Job drawing, mm, ordinate dimensions from the low corner. One solid piece. Round coordinates to 2 decimals unless told otherwise and drop trailing zeros. Loops run counter-clockwise (first coordinate to the right, second up) from the corner with the lowest first, then second, coordinate; pieces in that order, holes last. Notation, with made-up numbers: M 57,-17 L 77,-17 A23 ccw 77,-2 Z; hole C 79.5,52.5 d8. An arc over 180 degrees is marked long. Use a Markdown table: item, result. Add a question column.
(1) Two-plate mould, pull along X, no slides. Class the marked faces 1, 2 and 3: released by +X, released by -X, zero draft, split by the parting line, or undercut.
(2) Band-saw the part on D-D, the plane y = 50.5. Write the cut outline in (x, z).
(3) Wall check: L1, parallel to Y at x = 138.5, z = 4.5; L2, parallel to X at y = 198, z = 8; L3, parallel to X at y = 127, z = 12.25. Give the ranges that are in metal, low to high.
(4) Band-saw the part on A-A, the plane z = 8.5. Give the number of separate pieces and of enclosed holes in the cut face, and give its area (3 significant figures).
(5) Band-saw the part on C-C, the plane y = 127. Write the cut outline in (x, z), and give its area (3 significant figures).
(6) Band-saw the part on B-B, the plane x = 167. Write the cut outline in (y, z), and give its area (3 significant figures).
(7) Flat gauge pins, fed straight in: P1, Ø1.5, axis at y = 228, z = 7.5, coming from the +X side; P2, Ø6, axis at y = 242.5, z = 14.5, coming from the -X side; P3, Ø1, axis at y = 209, z = 14.5, coming from the +X side. Where does each tip first touch, or does it go through?
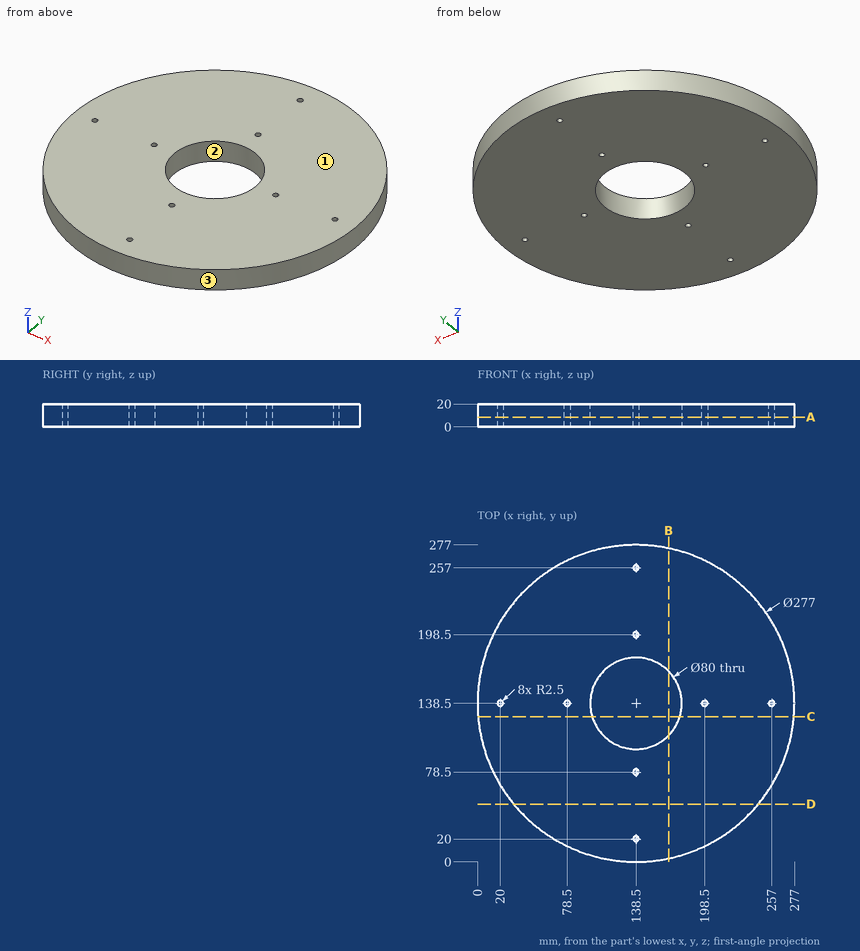
Return value:
| question | item | result |
|---|---|---|
| 1 | face 1 | zero draft |
| 1 | face 2 | undercut |
| 1 | face 3 | split by the parting line |
| 2 | outline | M 31.55,0 L 245.45,0 L 245.45,20 L 31.55,20 Z |
| 3 | L1 | 0 to 17.5, 22.5 to 76, 81 to 98.5, 178.5 to 196, 201 to 254.5, 259.5 to 277 |
| 3 | L2 | 13.43 to 136.05, 140.95 to 263.57 |
| 3 | L3 | 0.48 to 100.19, 176.81 to 276.52 |
| 4 | separate pieces | 1 |
| 4 | enclosed holes | 9 |
| 4 | area | 55,100 mm^2 |
| 5 | outline | M 0.48,0 L 100.19,0 L 100.19,20 L 0.48,20 Z; M 176.81,0 L 276.52,0 L 276.52,20 L 176.81,20 Z |
| 5 | area | 3,990 mm^2 |
| 6 | outline | M 2.96,0 L 110.43,0 L 110.43,20 L 2.96,20 Z; M 166.57,0 L 274.04,0 L 274.04,20 L 166.57,20 Z |
| 6 | area | 4,300 mm^2 |
| 7 | P1 | x = 244.83 |
| 7 | P2 | x = 43.73 |
| 7 | P3 | x = 258.01 |
